Design review of the part built by this model. Coordinates are the model's own, in mm. A direction names the side the tool comes from. Coordinates: 2 decimals unless noted, no trailing zeros. Order: outer loops, then holes, each group sorted by start corner. A loop starts at its lowest first (then second) coordinate and runs counter-clockwise, first axis right, second up. Notation, with made-up numbers: (-22.75, -18) -> (29.25, -18) arc R19 ccw to (29.25, -13) -> close; hole circle Ø8 at (75, 71). An arc over 180 degrees is marked (long way). Use a Markdown table: item, result. Add a question column.
Q1. Machinability: for faces 1 (the face through (16, -9, 5)), 2 (the face through (-20, 15, 5)), 3 (the face through (-16, -9, 5)), which of the approach directions +Z, -Z, +X, -X, +Y, -Y give a long, thin tool a straight path to every point of the face, cutting with its end or side? Answer none if there is none.
Q2. Insertion check: pin 1 (3 mm diameter, centred on y = -12, z = 5.5, fed in from -X); pin 2 (8 mm diameter, centred on x = 10.5, y = 13, fed in from -Z); pin 3 (4 mm diameter, centred on y = -5.5, z = 9.5, fed in from +X); pin 4 (3 mm diameter, centred on x = -23, y = -2, fed in from -Z). Each pin has a flat end and moves straight along its axis. Give the tip position at first contact, or say it passes through.
Q3. The part is to be moulded in two halves that separate along X. For faces 4 (the face through (-10, 21, 5)), 5 (the face through (-1.75, -9, 5)), 6 (the face through (-23, 0, 5)), 7 (the face through (30, 7, 5)), say which applies: pulls with the +X half, pulls with the -X half, needs draft (parallel to the pull), parting line crosses it, or undercut.
Q4. Add section D-D (y = -15). State the section outline as (x, z) points, then the cut area to 3 significant figures.
Q5. Add section B-B (y = 25). State the section outline as (x, z) points, then the cut area to 3 significant figures.
Q6. Wall thickness on probe 1 along X at (y, z) = (-14, 8.75); probe 2 along Z at (x, y) = (-13, 14); probe 3 along X at (y, z) = (27, 8.5): over which ranges is each line inside the solid? List them lowest first.
Q7. Add section A-A (z = 5). State the section outline as (x, y) points, then the cut area to 3 significant figures.
Q8. Add section C-C (x = -8). State the section outline as (y, z) points.
from build123d import *

# Parameters (mm, degrees)
F1_DEPTH = 10
F2_R     = 6.5
F2_R_2   = 2.5
F3_DEPTH = 10
F4_DEPTH = 12.5


with BuildPart() as f1:
    # F0 (on Top) → F1 (new body)
    with BuildSketch(Plane.XY):
        Polygon((-30, 15), (-30, 0), (-16, 0), (-16, -18), (-1.75, -18), (-1.75, 0), (0, 0), (1.75, 0), (1.75, -18), (16, -18), (16, 0), (30, 0), (30, 15), (10, 15), (10, 25), (0, 25), (-10, 25), (-10, 15), align=None)
    extrude(amount=F1_DEPTH)

    # F2 (on Right) → F3 (join, symmetric)
    with BuildSketch(Plane.YZ):
        with Locations((24.9999996855, 4.9974920324)):
            Circle(F2_R)
        with Locations((24.9999996855, 4.9974920324)):
            Circle(F2_R_2, mode=Mode.SUBTRACT)
    extrude(amount=F3_DEPTH, both=True)

    # F2 (on Right) → F4 (cut, symmetric)
    with BuildSketch(Plane.YZ):
        with Locations((24.9999996855, 4.9974920324)):
            Circle(F2_R_2)
    extrude(amount=F4_DEPTH, both=True, mode=Mode.SUBTRACT)


solid = f1.part
Established:
| question | item | result |
|---|---|---|
| 1 | face 1 | +Z, -Z, +X, -Y |
| 1 | face 2 | +Z, -Z, -X, +Y |
| 1 | face 3 | +Z, -Z, -X, -Y |
| 2 | pin 1 | x = -16 |
| 2 | pin 2 | z = 0 |
| 2 | pin 3 | x = 16 |
| 2 | pin 4 | through |
| 3 | face 4 | pulls with the -X half |
| 3 | face 5 | undercut |
| 3 | face 6 | needs draft |
| 3 | face 7 | pulls with the +X half |
| 4 | outline | (-16, 0) -> (-1.75, 0) -> (-1.75, 10) -> (-16, 10) -> close; (1.75, 0) -> (16, 0) -> (16, 10) -> (1.75, 10) -> close |
| 4 | area | 285 mm^2 |
| 5 | outline | (-10, -1.5) -> (10, -1.5) -> (10, 2.5) -> (-10, 2.5) -> close; (-10, 7.5) -> (10, 7.5) -> (10, 11.5) -> (-10, 11.5) -> close |
| 5 | area | 160 mm^2 |
| 6 | probe 1 | -16 to -1.75, 1.75 to 16 |
| 6 | probe 2 | 0 to 10 |
| 6 | probe 3 | -10 to 10 |
| 7 | outline | (-30, 0) -> (-16, 0) -> (-16, -18) -> (-1.75, -18) -> (-1.75, 0) -> (1.75, 0) -> (1.75, -18) -> (16, -18) -> (16, 0) -> (30, 0) -> (30, 15) -> (10, 15) -> (10, 22.5) -> (-10, 22.5) -> (-10, 15) -> (-30, 15) -> close; (-10, 27.5) -> (10, 27.5) -> (10, 31.5) -> (-10, 31.5) -> close |
| 7 | area | 1,640 mm^2 |
| 8 | outline | (-18, 0) -> (20.84, 0) arc R6.5 ccw (long way) to (20.85, 10) -> (-18, 10) -> close; hole circle Ø5 at (25, 5) |
